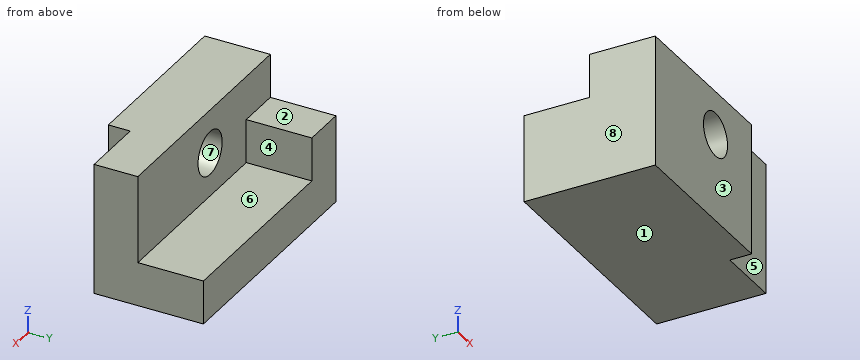
```python
from build123d import *

# Parameters (mm, degrees)
BOSS_EXTRUDE1_START     = -12.7
BOSS_EXTRUDE1_DEPTH     = 76.2
BOSS_EXTRUDE2_START     = -50.8
BOSS_EXTRUDE2_DEPTH     = 38.1
SKETCH7_R               = 12.7
CUT_EXTRUDE1_DEPTH      = 257.841604885
CUT_EXTRUDE2_DEPTH      = 262.509005581
CUT_EXTRUDE2_DEPTH_BACK = 262.509005581


with BuildPart() as part:
    # Sketch5 → Boss-Extrude1 (new body)
    with BuildSketch(Plane(origin=(0, 114.3, 0), x_dir=(-1, 0, 0), z_dir=(0, 1, 0)).offset(BOSS_EXTRUDE1_START)):
        Polygon((-88.9, -25.4), (-88.9, -76.2), (-228.6, -76.2), (-228.6, -50.8), (-114.3, -50.8), (-114.3, -25.4), align=None)
    extrude(amount=-BOSS_EXTRUDE1_DEPTH)

    # Sketch6 → Boss-Extrude2 (add)
    with BuildSketch(Plane(origin=(0, 114.3, 0), x_dir=(-1, 0, 0), z_dir=(0, 1, 0)).offset(BOSS_EXTRUDE2_START)):
        Polygon((-228.6, 0), (-88.9, 0), (-88.9, -25.4), (-114.3, -25.4), (-114.3, -50.8), (-228.6, -50.8), align=None)
    extrude(amount=-BOSS_EXTRUDE2_DEPTH)

    # Sketch7 → Cut-Extrude1 (cut, through all)
    with BuildSketch(Plane(origin=(0, 114.3, 0), x_dir=(-1, 0, 0), z_dir=(0, 1, 0))):
        with Locations(Location((-152.4, -25.4, 0), (0, 0, 90))):
            Circle(SKETCH7_R)
    extrude(amount=-CUT_EXTRUDE1_DEPTH, mode=Mode.SUBTRACT)

    # Sketch8 → Cut-Extrude2 (cut, two sides: drawn at the far end of the back side and taken through both)
    with BuildSketch(Plane.XY.offset(-CUT_EXTRUDE2_DEPTH_BACK)):
        Polygon((545.509367729, 38.1), (228.6, 38.1), (190.5, 38.1), (190.5, 25.4), (190.5, -291.509367729), (621.753014004, -755.995134283), (976.762381733, -426.385766553), align=None)
    extrude(amount=CUT_EXTRUDE2_DEPTH + CUT_EXTRUDE2_DEPTH_BACK, mode=Mode.SUBTRACT)


solid = part.part
```
The listing builds one solid part. Answer for the finished solid, in the listing's coordinates (mm). Face numbers are marked on the shaded views. A direction names the side the tool comes from. Coordinates: 2 decimals unless noted, no trailing zeros. Write each loop counter-clockwise with the first axis right and the second up, starting at its lowest first coordinate (ties: lowest second). Pieces come first, ordered by that corner, then holes. Notation, with made-up numbers: M 64,54.25 L 109,54.25 A18 cw 109,89.25 Z; hole C 43,31 d8. An arc over 180 degrees is marked long. Use a Markdown table: item, result. Add a question column.
1. Section A-A (x = 152.4) is taken. Give the vertices of the cut face in (y, z).
2. For a pull along X with two mould halves and no side action, classify the marked faces 6, 7 and 8 as +X half, -X half, draft (parallel to the pull), parting line (faces both ways), or undercut.
3. Given P1, Ø10, axis at y = 29, z = -33.5, coming from the +X side; P2, Ø10, axis at y = 91.5, z = -41, coming from the +X side; P3, Ø23, axis at x = 152.4, z = -25.4, coming from the -Y side; P4, Ø5, axis at x = 113.5, y = 92.5, coming from the +Z side, each flat-ended and moving along its own axis, determine where each tip first touches the part or whether it passes through.
4. Section C-C (y = 47.5) is taken. Give the vertices of the cut face in (x, z).
5. Which of the six approach directions +Z, -Z, +X, -X, +Y, -Y give full straight-line access (tool end or side, diameter ignored) to the marked faces 1, 2, 3, 4 and 5?
6. Section B-B (z = -10) is taken. Give the vertices of the cut face in (x, y).
7. Section D-D (x = 174.5) is taken. Give the vertices of the cut face in (y, z), plus the area to 3 significant figures.
8. Straight lines are drawn through the part: line 1 along X through (y, z) = (44, -25); line 2 along Z through (x, y) = (152, 42); line 3 along X through (y, z) = (36, -25.4). For each, find the intervals that lie inside material, in ascending order. Write a range as [from, to].
Data:
| question | item | result |
|---|---|---|
| 1 | outline | M 25.4,-76.2 L 101.6,-76.2 L 101.6,-50.8 L 63.5,-50.8 L 63.5,-38.1 L 25.4,-38.1 Z; M 25.4,-12.7 L 63.5,-12.7 L 63.5,0 L 25.4,0 Z |
| 2 | face 6 | draft |
| 2 | face 7 | undercut |
| 2 | face 8 | -X half |
| 3 | P1 | stops at x = 190.5 |
| 3 | P2 | stops at x = 114.3 |
| 3 | P3 | passes through |
| 3 | P4 | stops at z = -25.4 |
| 4 | outline | M 88.9,-76.2 L 228.6,-76.2 L 228.6,0 L 88.9,0 Z; hole C 152.4,-25.4 d25.4 |
| 5 | face 1 | -Z, +X, -X, +Y, -Y |
| 5 | face 2 | +Z, +X, -X, +Y |
| 5 | face 3 | +Z, -Z, +X, -X, -Y |
| 5 | face 4 | +Z, +X, +Y |
| 5 | face 5 | +Z, -Z, +X, -Y |
| 6 | outline | M 88.9,25.4 L 190.5,25.4 L 190.5,38.1 L 228.6,38.1 L 228.6,63.5 L 88.9,63.5 Z |
| 7 | outline | M 25.4,-76.2 L 101.6,-76.2 L 101.6,-50.8 L 63.5,-50.8 L 63.5,0 L 25.4,0 Z |
| 7 | area | 3,870 mm2 |
| 8 | line 1 | x = [88.9, 139.71], [165.09, 228.6] |
| 8 | line 2 | z = [-76.2, -38.09], [-12.71, 0] |
| 8 | line 3 | x = [88.9, 139.7], [165.1, 190.5] |
